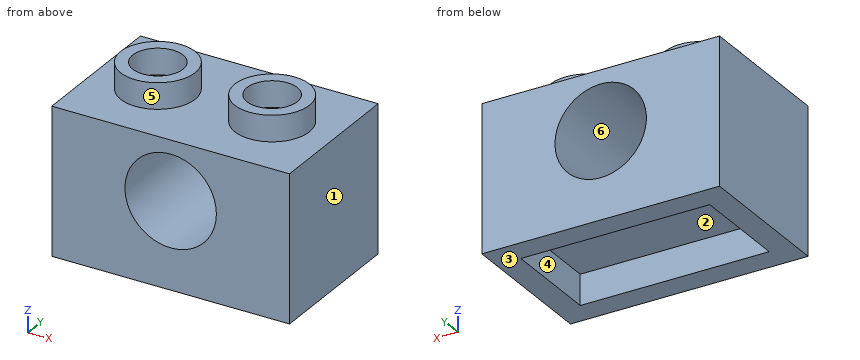
from build123d import *

# Parameters (mm, degrees)
F1_START = 10
F0_W     = 15.6
F0_H     = 9.6
F0_R     = 3
F1_DEPTH = 9.7
F2_R     = 2.45
F2_R_2   = 1.65
F3_DEPTH = 1.7
F5_DEPTH = 2
F0_R_2   = 2.3
F6_DEPTH = 0.8
F7_R     = 3
F7_R_2   = 2.3
F8_DEPTH = 0.8


with BuildPart() as f1:
    # F0 (on Front) → F1 (new body)
    with BuildSketch(Plane.XZ.offset(F1_START)):
        with Locations((-5.3637987003, 2.2607615549)):
            Rectangle(F0_W, F0_H)
        with Locations((-5.3637987003, 3.1607615549)):
            Circle(F0_R, mode=Mode.SUBTRACT)
    extrude(amount=F1_DEPTH)

    # F2 (on face) → F3 (join)
    with BuildSketch(Plane.XY.offset(7.0607615549)):
        with Locations((-1.6137987003, -14.85)):
            Circle(F2_R)
        with Locations((-1.6137987003, -14.85)):
            Circle(F2_R_2, mode=Mode.SUBTRACT)
        with Locations((-9.1137987003, -14.85)):
            Circle(F2_R)
        with Locations((-9.1137987003, -14.85)):
            Circle(F2_R_2, mode=Mode.SUBTRACT)
    extrude(amount=F3_DEPTH)

    # F4 (on face) → F5 (cut)
    with BuildSketch(Plane(origin=(0, 0, -2.5392384451), x_dir=(1, 0, 0), z_dir=(0, 0, -1))):
        Polygon((-11.5637987003, 18.1), (-11.5637987003, 14.85), (-11.5637987003, 11.6), (-5.3637987003, 11.6), (0.8362012997, 11.6), (0.8362012997, 14.85), (0.8362012997, 18.1), (-5.3637987003, 18.1), align=None)
    extrude(amount=-F5_DEPTH, mode=Mode.SUBTRACT)

    # F0 (on Front) → F6 (cut)
    with BuildSketch(Plane.XZ):
        with Locations((-5.3637987003, 3.1607615549)):
            Circle(F0_R)
        with Locations((-5.3637987003, 3.1607615549)):
            Circle(F0_R_2, mode=Mode.SUBTRACT)
    extrude(amount=F6_DEPTH, mode=Mode.SUBTRACT)

    # F7 (on face) → F8 (cut)
    with BuildSketch(Plane.XZ.offset(19.7)):
        with Locations((-5.3637987003, 3.1607615549)):
            Circle(F7_R)
        with Locations((-5.3637987003, 3.1607615549)):
            Circle(F7_R_2, mode=Mode.SUBTRACT)
    extrude(amount=-F8_DEPTH, mode=Mode.SUBTRACT)


solid = f1.part
Can you work these out from the model? Positions are in its coordinate system, mm. Face numbers are marked on the shaded views. A direction names the side the tool comes from. Coordinates: 2 decimals unless noted, no trailing zeros. Order: outer loops, then holes, each group sorted by start corner. A loop starts at its lowest first (then second) coordinate and runs counter-clockwise, first axis right, second up. Notation, with made-up numbers: (-3, 85) - (51, 85) arc R25 cw to (51, 119) - close; hole circle Ø8 at (-11, 3). An arc over 180 degrees is marked (long way). Answer as a JSON object with one key per item and string values. Group by question number.
Q1. Imagine slicing it at B-B (y = -13.5). Please give me the cut outline in (x, z), and give its area (3 significant figures).
Q2. Imagine slicing it at A-A (z = -2). Please give me the cut outline in (x, y), and give its area (3 significant figures).
Q3. On a 3-axis mill with a long thin cutter (end or side, diameter ignored), from which of +Z, -Z, +X, -X, +Y, -Y can I reach the whole of each face in a straight line? I mean the marked faces 4, 5 and 6. Say none if no direction works.
Q4. Imagine slicing it at C-C (x = -5.75). Please give me the cut outline in (y, z), and give its area (3 significant figures).
Q5. We'd pull the mould along X, two halves only. Please class the marked faces 1, 2 and 3: +X half, -X half, draft (parallel to the pull), parting line (faces both ways), or undercut.
Q6. Will these pins go through, and if not, where does the flat tip stop? P1, Ø2, axis at x = -9.11, y = -14.85, coming from the +Z side; P2, Ø4, axis at x = -1.61, y = -14.85, coming from the -Z side.
Q7. I need wall thicknesses on line 1 (X direction, y = -15.25, z = 7.75); line 2 (X direction, y = -18, z = -0.75); line 3 (Z direction, x = -0.25, y = -12.75). Which ranges of each line are inside material? Lowest first, please. Write a range as from..to.
Q8. Imagine slicing it at D-D (x = -1.25). Please give me the cut outline in (y, z).
Determined:
{
 "1": {"outline": "(-13.16, -2.54) - (-11.56, -2.54) - (-11.56, -0.54) - (0.84, -0.54) - (0.84, -2.54) - (2.44, -2.54) - (2.44, 7.06) - (0.43, 7.06) - (0.43, 8.76) - (-0.67, 8.76) - (-0.67, 7.06) - (-2.56, 7.06) - (-2.56, 8.76) - (-3.66, 8.76) - (-3.66, 7.06) - (-7.07, 7.06) - (-7.07, 8.76) - (-8.17, 8.76) - (-8.17, 7.06) - (-10.06, 7.06) - (-10.06, 8.76) - (-11.16, 8.76) - (-11.16, 7.06) - (-13.16, 7.06) - close; hole circle Ø6 at (-5.36, 3.16)", "area": "104 mm2"},
 "2": {"outline": "(-13.16, -19.7) - (2.44, -19.7) - (2.44, -10) - (-13.16, -10) - close; hole (-11.56, -18.1) - (0.84, -18.1) - (0.84, -11.6) - (-11.56, -11.6) - close", "area": "70.7 mm2"},
 "3": {"face 4": "-Z", "face 5": "+Z", "face 6": "+Y, -Y"},
 "4": {"outline": "(-19.7, -2.54) - (-18.1, -2.54) - (-18.1, -0.54) - (-11.6, -0.54) - (-11.6, -2.54) - (-10, -2.54) - (-10, 0.19) - (-19.7, 0.19) - close; (-19.7, 6.14) - (-10, 6.14) - (-10, 7.06) - (-19.7, 7.06) - close", "area": "22.4 mm2"},
 "5": {"face 1": "+X half", "face 2": "undercut", "face 3": "draft"},
 "6": {"P1": "stops at z = 7.06", "P2": "stops at z = -0.54"},
 "7": {"line 1": "x = -11.53..-10.71, -7.51..-6.7, -4.03..-3.21, -0.01..0.8", "line 2": "x = -13.16..-11.56, 0.84..2.44", "line 3": "z = -0.54..7.06"},
 "8": {"outline": "(-19.7, -2.54) - (-18.1, -2.54) - (-18.1, -0.54) - (-11.6, -0.54) - (-11.6, -2.54) - (-10, -2.54) - (-10, 7.06) - (-12.43, 7.06) - (-12.43, 8.76) - (-13.24, 8.76) - (-13.24, 7.06) - (-16.46, 7.06) - (-16.46, 8.76) - (-17.27, 8.76) - (-17.27, 7.06) - (-19.7, 7.06) - close"}
}
